Here's how the part is built. I have some questions about the finished solid (model axes, mm). Face numbers are marked on the shaded views. A direction names the side the tool comes from. Round coordinates to 2 decimals unless told otherwise and drop trailing zeros. Loops run counter-clockwise (first coordinate to the right, second up) from the corner with the lowest first, then second, coordinate; pieces in that order, holes last. Notation, with made-up numbers: M 37.25,55 L 49.25,55 A18 cw 49.25,76 Z; hole C -32,52.5 d11. An arc over 180 degrees is marked long. Answer as CSV lines item,"result".
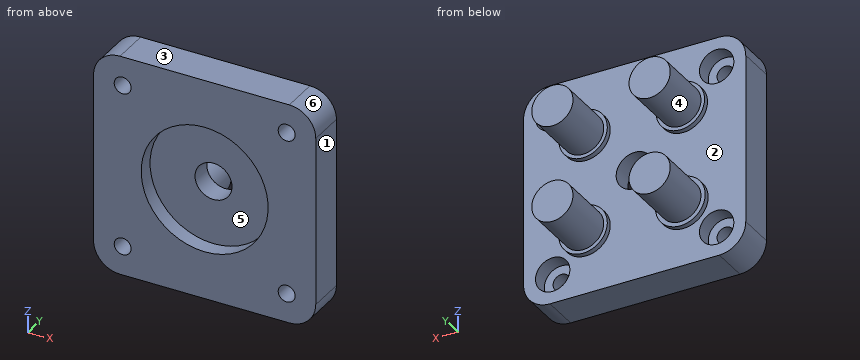
```python
from build123d import *

# Parameters (mm, degrees)
SKIZZE1_W                       = 42
SKIZZE1_H                       = 42
SKIZZE1_R                       = 1.6
SKIZZE1_R_2                     = 3.5
AUFSATZ_LINEAR_AUSTRAGEN1_DEPTH = 7
SKIZZE2_R                       = 3.9
AUFSATZ_LINEAR_AUSTRAGEN2_DEPTH = 11.4
VERRUNDUNG1_R                   = 5
SKIZZE3_R                       = 12
SCHNITT_LINEAR_AUSTRAGEN1_DEPTH = 3
SKIZZE4_R                       = 3.25
SCHNITT_LINEAR_AUSTRAGEN2_DEPTH = 3
SKIZZE5_R                       = 4.7
SKIZZE5_R_2                     = 4.580495264
AUFSATZ_LINEAR_AUSTRAGEN3_DEPTH = 1


with BuildPart() as part:
    # Skizze1 → Aufsatz-Linear austragen1 (new body)
    with BuildSketch(Plane(origin=(0, 0, 0), x_dir=(1, 0, 0), z_dir=(0, 1, 0))):
        with Locations((21, 21)):
            Rectangle(SKIZZE1_W, SKIZZE1_H)
        with Locations(Location((5.5, 36.5, 0), (0, 0, 270))):
            Circle(SKIZZE1_R, mode=Mode.SUBTRACT)
        with Locations(Location((36.5, 36.5, 0), (0, 0, 270))):
            Circle(SKIZZE1_R, mode=Mode.SUBTRACT)
        with Locations(Location((5.5, 5.5, 0), (0, 0, 270))):
            Circle(SKIZZE1_R, mode=Mode.SUBTRACT)
        with Locations(Location((36.5, 5.5, 0), (0, 0, 270))):
            Circle(SKIZZE1_R, mode=Mode.SUBTRACT)
        with Locations(Location((21, 21, 0), (0, 0, 270))):
            Circle(SKIZZE1_R_2, mode=Mode.SUBTRACT)
    extrude(amount=AUFSATZ_LINEAR_AUSTRAGEN1_DEPTH)

    # Skizze2 → Aufsatz-Linear austragen2 (add)
    with BuildSketch(Plane(origin=(0, 7, 0), x_dir=(1, 0, 0), z_dir=(0, 1, 0))):
        with Locations(Location((11.807611845, 30.192388155, 0), (0, 0, 90))):
            Circle(SKIZZE2_R)
        with Locations(Location((30.192388155, 30.192388155, 0), (0, 0, 90))):
            Circle(SKIZZE2_R)
        with Locations(Location((30.192388155, 11.807611845, 0), (0, 0, 90))):
            Circle(SKIZZE2_R)
        with Locations(Location((11.807611845, 11.807611845, 0), (0, 0, 90))):
            Circle(SKIZZE2_R)
    extrude(amount=AUFSATZ_LINEAR_AUSTRAGEN2_DEPTH)

    # Verrundung1
    verrundung1_edges = [part.edges().sort_by_distance(p)[0] for p in [
        (0, 3.5, -42),
        (42, 3.5, -42),
        (42, 3.5, 0),
        (0, 3.5, 0),
    ]]
    fillet(verrundung1_edges, radius=VERRUNDUNG1_R)

    # Skizze3 → Schnitt-Linear austragen1 (cut)
    with BuildSketch(Plane.XZ):
        with Locations(Location((21, -21, 0), (0, 0, 270))):
            Circle(SKIZZE3_R)
    extrude(amount=-SCHNITT_LINEAR_AUSTRAGEN1_DEPTH, mode=Mode.SUBTRACT)

    # Skizze4 → Schnitt-Linear austragen2 (cut)
    with BuildSketch(Plane(origin=(0, 7, 0), x_dir=(1, 0, 0), z_dir=(0, 1, 0))):
        with Locations(Location((5.5, 36.5, 0), (0, 0, 270))):
            Circle(SKIZZE4_R)
        with Locations(Location((36.5, 36.5, 0), (0, 0, 270))):
            Circle(SKIZZE4_R)
        with Locations(Location((5.5, 5.5, 0), (0, 0, 270))):
            Circle(SKIZZE4_R)
        with Locations(Location((36.5, 5.5, 0), (0, 0, 270))):
            Circle(SKIZZE4_R)
    extrude(amount=-SCHNITT_LINEAR_AUSTRAGEN2_DEPTH, mode=Mode.SUBTRACT)

    # Skizze5 → Aufsatz-Linear austragen3 (add)
    with BuildSketch(Plane(origin=(0, 7, 0), x_dir=(1, 0, 0), z_dir=(0, 1, 0))):
        with Locations(Location((11.807611845, 30.192388155, 0), (0, 0, 90))):
            Circle(SKIZZE5_R)
        with Locations(Location((11.807611845, 11.807611845, 0), (0, 0, 90))):
            Circle(SKIZZE5_R_2)
        with Locations(Location((30.192388155, 11.807611845, 0), (0, 0, 90))):
            Circle(SKIZZE5_R_2)
        with Locations(Location((30.192388155, 30.192388155, 0), (0, 0, 90))):
            Circle(SKIZZE5_R_2)
    extrude(amount=AUFSATZ_LINEAR_AUSTRAGEN3_DEPTH)


solid = part.part
```
1. For P1, Ø8.5, axis at x = 36.5, z = -5.5, coming from the +Y side; P2, Ø4, axis at x = 32.5, y = 11.5, coming from the +Z side; P3, Ø4, axis at x = 5.5, z = -5.5, coming from the +Y side, each with a flat end and sliding along its axis, tell me the tip position at first contact or that it passes through.
Evaluation:
P1,"stops at y = 7"
P2,"stops at z = -7.92"
P3,"stops at y = 4"
2. Which directions (+Z, -Z, +X, -X, +Y, -Y) give clear straight access to the entire face, cutting with the end or side of a thin tool? Please do the marked faces 4, 5 and 6.
Evaluation:
face 4,"+Y"
face 5,"-Y"
face 6,"+Z, +X, +Y, -Y"
3. We'd pull the mould along Z, two halves only. Please class the marked faces 1, 2 and 3: pulls with the +Z half, pulls with the -Z half, needs draft (parallel to the pull), parting line crosses it, or undercut.
Evaluation:
face 1,"needs draft"
face 2,"undercut"
face 3,"pulls with the +Z half"
4. I want a section at A-A, the plane x = 5.5. Please give me the cut outline in (y, z).
Evaluation:
outline,"M 0,-42 L 7,-42 L 7,-39.75 L 4,-39.75 L 4,-38.1 L 0,-38.1 Z; M 0,-34.9 L 4,-34.9 L 4,-33.25 L 7,-33.25 L 7,-8.75 L 4,-8.75 L 4,-7.1 L 0,-7.1 Z; M 0,-3.9 L 4,-3.9 L 4,-2.25 L 7,-2.25 L 7,0 L 0,0 Z"
5. I want a section at D-D, the plane z = -21. Please give me the cut outline in (x, y), and give its area (3 significant figures).
Evaluation:
outline,"M 0,0 L 9,0 L 9,3 L 17.5,3 L 17.5,7 L 0,7 Z; M 24.5,3 L 33,3 L 33,0 L 42,0 L 42,7 L 24.5,7 Z"
area,"194 mm²"
6. I want a section at B-B, the plane z = -5.5. Please give me the cut outline in (x, y), and give its area (3 significant figures).
Evaluation:
outline,"M 0,0 L 3.9,0 L 3.9,4 L 2.25,4 L 2.25,7 L 0,7 Z; M 7.1,0 L 34.9,0 L 34.9,4 L 33.25,4 L 33.25,7 L 8.75,7 L 8.75,4 L 7.1,4 Z; M 38.1,0 L 42,0 L 42,7 L 39.75,7 L 39.75,4 L 38.1,4 Z"
area,"229 mm²"
7. I want a section at C-C, the plane x = 21. Please give me the cut outline in (y, z).
Evaluation:
outline,"M 0,-42 L 7,-42 L 7,-24.5 L 3,-24.5 L 3,-33 L 0,-33 Z; M 0,-9 L 3,-9 L 3,-17.5 L 7,-17.5 L 7,0 L 0,0 Z"
8. If I drill on line 1 (Z direction, x = 36.5, y = 0.95); line 2 (X direction, y = 2.85, z = -36.5); line 3 (X direction, y = 5.35, z = -36.5), over which ranges is the centre line in solid material (lowest first)? Write a range as [from, to].
Evaluation:
line 1,"z = [-42, -38.1], [-34.9, -7.1], [-3.9, 0]"
line 2,"x = [0, 3.9], [7.1, 34.9], [38.1, 42]"
line 3,"x = [0, 2.25], [8.75, 33.25], [39.75, 42]"
